from build123d import *

# Parameters (mm, degrees)
SKETCH1_R               = 3
BOSS_EXTRUDE1_DEPTH     = 9.8
CUT_EXTRUDE1_DEPTH      = 18.205812971
CUT_EXTRUDE1_DEPTH_BACK = 18.205812971
CHAMFER1_SIZE           = 0.5


with BuildPart() as part:
    # Sketch1 → Boss-Extrude1 (new, symmetric)
    with BuildSketch(Plane(origin=(0, 0, 0), x_dir=(0, 0, -1), z_dir=(1, 0, 0))):
        Polygon((-10, 10), (-10, -10), (10, -10), (10, 10), (7.5, 10), (6, 8.5), (4.5, 10), (1.5, 10), (0, 8.5), (-1.5, 10), (-4.5, 10), (-6, 8.5), (-7.5, 10), align=None)
        Circle(SKETCH1_R, mode=Mode.SUBTRACT)
    extrude(amount=BOSS_EXTRUDE1_DEPTH, both=True)

    # Sketch2 → Cut-Extrude1 (cut, two sides: drawn at the far end of the back side and taken through both)
    with BuildSketch(Plane.XY.offset(-CUT_EXTRUDE1_DEPTH_BACK)):
        Polygon((-7.5, 10), (-4.5, 10), (-6, 8.5), align=None)
        Polygon((0, 8.5), (-1.5, 10), (1.5, 10), align=None)
        Polygon((4.5, 10), (6, 8.5), (7.5, 10), align=None)
    extrude(amount=CUT_EXTRUDE1_DEPTH + CUT_EXTRUDE1_DEPTH_BACK, mode=Mode.SUBTRACT)

    # Chamfer1
    chamfer1_edges = [part.edges().sort_by_distance(p)[0] for p in [
        (-9.8, 0, 3),
        (9.8, 0, 3),
    ]]
    chamfer(chamfer1_edges, length=CHAMFER1_SIZE)


solid = part.part
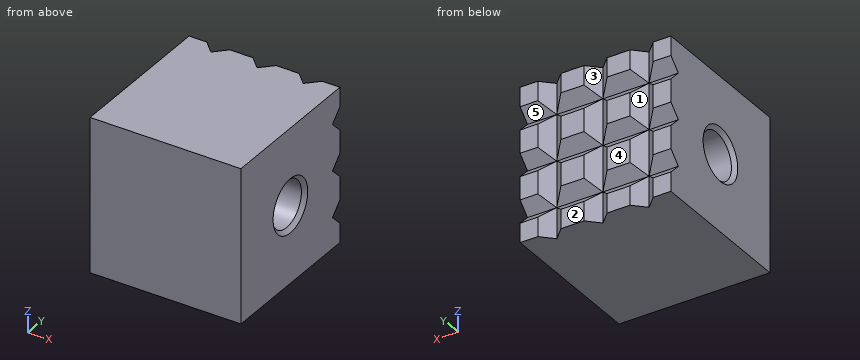
Source: CAD feature listing. Evaluate the final solid. Frame: model axes, mm. Face numbers are marked on the shaded views. A direction names the side the tool comes from. Give positions to 0.01 mm unless a question says otherwise; leave off trailing zeros. Write each loop counter-clockwise with the first axis right and the second up, starting at its lowest first coordinate (ties: lowest second). Pieces come first, ordered by that corner, then holes. Notation, with made-up numbers: M -27,-8.75 L -20,-8.75 A12 cw -20,10.25 Z; hole C -30.75,78 d8. An arc over 180 degrees is marked long. Return JSON: item names as keys, results as strings. Group by question number.
1) Cut plane A-A, the plane x = -1. Output: boundary loops of the cut face in (y, z), then the cut area to 3 significant figures.
2) Draft query along X for the marked faces 1 and 2. Return one class per face: released by +X, released by -X, zero draft, split by the parting line, or undercut.
3) Cut plane B-B, the plane y = 0. Output: boundary loops of the cut face in (x, z), then the cut area to 3 significant figures.
4) Ray query, L1, parallel to Z at x = -3.5, y = -2; L2, parallel to Y at x = -1.75, z = 0.75; L3, parallel to Y at x = -1.25, z = 6.5. Return the intervals inside material, ascending.
5) Set-up query: the marked faces 3, 4 and 5. Return all of +Z, -Z, +X, -X, +Y, -Y with unobstructed straight access to the full face (end or side cutting, diameter ignored); none if empty.
Data:
{
 "1": {"outline": "M -10,-10 L 9.5,-10 L 9.5,-7 L 8.5,-6 L 9.5,-5 L 9.5,-1 L 8.5,0 L 9.5,1 L 9.5,5 L 8.5,6 L 9.5,7 L 9.5,10 L -10,10 Z; hole C 0,0 d6", "area": "359 mm²"},
 "2": {"face 1": "undercut", "face 2": "zero draft"},
 "3": {"outline": "M -9.8,-10 L 9.8,-10 L 9.8,-3.5 L 9.3,-3 L -9.3,-3 L -9.8,-3.5 Z; M -9.8,3.5 L -9.3,3 L 9.3,3 L 9.8,3.5 L 9.8,10 L -9.8,10 Z", "area": "274 mm²"},
 "4": {"L1": "z = -10 to -2.24, 2.24 to 10", "L2": "y = -10 to -2.9, 2.9 to 9.25", "L3": "y = -10 to 9"},
 "5": {"face 3": "+Z, -Z, +Y", "face 4": "+Z, -Z, +X, -X, +Y", "face 5": "+X, -X, +Y"}
}
